```python
from build123d import *

# Parameters (mm, degrees)
BOSS_EXTRUDE1_DEPTH     = 20
CUT_EXTRUDE1_DEPTH      = 1
CUT_EXTRUDE1_DEPTH_BACK = 10
CUT_EXTRUDE2_DEPTH      = 10
CUT_EXTRUDE3_REACH      = 12


with BuildPart() as part:
    # Sketch1 → Boss-Extrude1 (new body, symmetric)
    with BuildSketch(Plane.XY):
        Polygon((-4.511794911, -6.86440678), (15.488205089, -6.86440678), (15.488205089, 8.13559322), (25.488205089, 8.13559322), (25.488205089, -16.86440678), (-24.511794911, -16.86440678), (-24.511794911, -6.86440678), align=None)
        Polygon((10.488205089, 8.13559322), (-4.511794911, -6.86440678), (15.488205089, -6.86440678), (15.488205089, 8.13559322), align=None)
    extrude(amount=BOSS_EXTRUDE1_DEPTH, both=True)

    # Sketch2 → Cut-Extrude1 (cut, two sides)
    with BuildSketch(Plane.XY.offset(20)) as cut_extrude1_sk:
        Polygon((-4.511794911, -6.86440678), (15.488205089, -6.86440678), (15.488205089, 8.13559322), (10.488205089, 8.13559322), align=None)
    extrude(amount=CUT_EXTRUDE1_DEPTH, mode=Mode.SUBTRACT)
    extrude(cut_extrude1_sk.sketch, amount=-CUT_EXTRUDE1_DEPTH_BACK, mode=Mode.SUBTRACT)

    # Sketch3 → Cut-Extrude2 (cut)
    with BuildSketch(Plane(origin=(0, 0, -20), x_dir=(-1, 0, 0), z_dir=(0, 0, -1))):
        Polygon((4.511794911, -6.86440678), (-15.488205089, -6.86440678), (-15.488205089, 8.13559322), (-10.488205089, 8.13559322), align=None)
    extrude(amount=-CUT_EXTRUDE2_DEPTH, mode=Mode.SUBTRACT)

    # Sketch4 → Cut-Extrude3 (cut, up to next)
    with BuildSketch(Plane(origin=(0, -6.86440678, 0), x_dir=(1, 0, 0), z_dir=(0, 1, 0)), mode=Mode.PRIVATE) as cut_extrude3_sk1:
        with BuildLine():
            Line((-24.511794911, 15), (-24.511794911, -15))
            ThreePointArc((-24.511794911, -15), (-9.511794911, 0), (-24.511794911, 15))
        make_face()
    cut_extrude3_tool1 = extrude(cut_extrude3_sk1.sketch, amount=-CUT_EXTRUDE3_REACH, mode=Mode.PRIVATE) & part.part
    add(cut_extrude3_tool1.solids().sort_by_distance((-18.145597, -6.864407, 0))[0], mode=Mode.SUBTRACT)


solid = part.part
```
The listing builds one solid part. Answer for the finished solid, in the listing's coordinates (mm). A direction names the side the tool comes from. Give positions to 0.01 mm unless a question says otherwise; leave off trailing zeros. Order: outer loops, then holes, each group sorted by start corner. A loop starts at its lowest first (then second) coordinate and runs counter-clockwise, first axis right, second up.
Item 1: Which of the six approach directions +Z, -Z, +X, -X, +Y, -Y give full straight-line access (tool end or side, diameter ignored) to faces 1 (the face through (-9, -6.864, 0)), 2 (the face through (6, -16.864, 0)), 3 (the face through (8, -1, -10)), 4 (the face through (8, -1, 10))?
From the geometry:
face 1: -X, +Y
face 2: +Z, -Z, +X, -X, -Y
face 3: -Z, -X, +Y
face 4: +Z, -X, +Y
Item 2: Given pin 1 Ø6 at (x, z) = (-1.5, -7) entering from +Y; pin 2 Ø8 at (y, z) = (3, 13) entering from -X; pin 3 Ø10 at (x, z) = (-9, 8) entering from +Y, each flat-ended and moving along its own axis, determine where each tip first touches the part or whether it passes through.
From the geometry:
pin 1: stops at y = -0.85
pin 2: stops at x = 2.71
pin 3: stops at y = -6.35
Item 3: The part is cut by section A-A, the plane x = -19. Give the vertices of the cut face in (y, z).
From the geometry:
outline: (-16.86, -20) - (-6.86, -20) - (-6.86, -13.95) - (-16.86, -13.95) - close; (-16.86, 13.95) - (-6.86, 13.95) - (-6.86, 20) - (-16.86, 20) - close
Item 4: Find the intervals of material crossed by probe 1 along X at (y, z) = (-6.5, 14); probe 2 along Y at (x, z) = (-5, -8); probe 3 along Z at (x, y) = (-18, -11.25), in increasing order.
From the geometry:
probe 1: x = 15.49 to 25.49
probe 2: y = -16.86 to -6.86
probe 3: z = -20 to -13.51, 13.51 to 20
Item 5: The part is cut by section B-B, the plane z = 0. Give the vertices of the cut face in (x, y).
From the geometry:
outline: (-9.51, -16.86) - (25.49, -16.86) - (25.49, 8.14) - (10.49, 8.14) - (-4.51, -6.86) - (-9.51, -6.86) - close
Item 6: The part is cut by section C-C, the plane y = -3.5. Give the vertices of the cut face in (x, z), and give its area (3 significant figures).
From the geometry:
outline: (-1.15, -10) - (15.49, -10) - (15.49, -20) - (25.49, -20) - (25.49, 20) - (15.49, 20) - (15.49, 10) - (-1.15, 10) - close
area: 733 mm2
Item 7: The part is cut by section D-D, the plane x = -14. Give the vertices of the cut face in (y, z), and give its area (3 significant figures).
From the geometry:
outline: (-16.86, -20) - (-6.86, -20) - (-6.86, -10.7) - (-16.86, -10.7) - close; (-16.86, 10.7) - (-6.86, 10.7) - (-6.86, 20) - (-16.86, 20) - close
area: 186 mm2
